Study the drawing (mm; zero at the part's minimum x, y, z) and answer. A direction names the side the tool comes from. Coordinates: 2 decimals unless noted, no trailing zeros. Order: outer loops, then holes, each group sorted by start corner. A loop starts at its lowest first (then second) coordinate and runs counter-clockwise, first axis right, second up. Notation, with made-up numbers: M 81,22.25 L 87,22.25 A14 ccw 87,46.25 Z; hole C 25,59.25 d2. An arc over 180 degrees is marked long. Use a Markdown table: item, result. Add a question column.
1) For the marked faces 1 and 2, determine the directions among +Z, -Z, +X, -X, +Y, -Y from which every point of the face is accessible in a straight line to the end or side of a thin tool.
2) Find section A-A on z = 14.5. Write down the section's boundary in (x, y) (1 decimal).
3) Find the intervals of material crossed by probe 1 along Y at (x, z) = (21, 4.5); probe 2 along X at (y, z) = (36.5, 2.25); probe 3 along Y at (x, z) = (11.5, 18.5), in increasing order. Write a range as [from, to].
4) Each of these flat-tipped pins is pushed along its axis until it touches: pin 1 Ø1.5 at (x, z) = (6.5, 3.5) entering from -Y (1 decimal); pin 2 Ø1.7 at (x, z) = (10, 9.5) entering from +Y; pin 3 Ø4 at (y, z) = (5.5, 17) entering from -X. Where does it stop, or does it pass through?
5) Find section B-B on x = 10. Write down the section's boundary in (y, z).
6) Find section C-C on y = 25.5. Write down the section's boundary in (x, z).
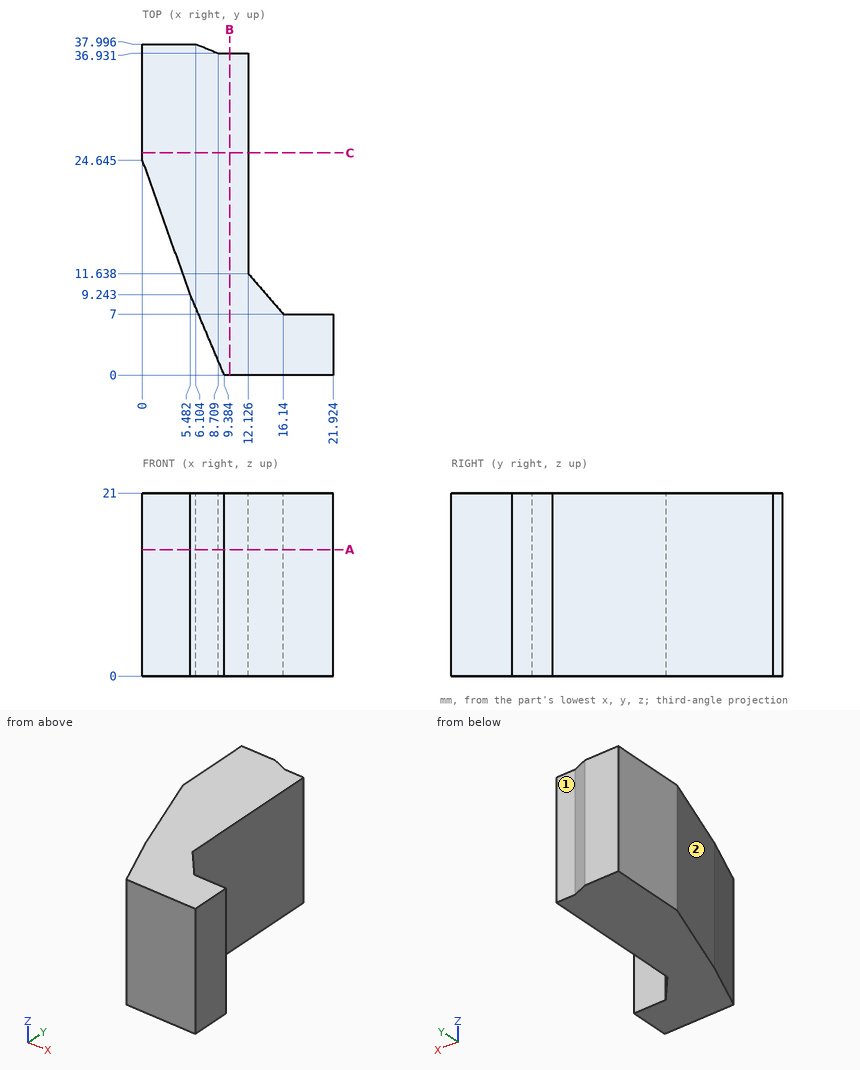
Check result:
| question | item | result |
|---|---|---|
| 1 | face 1 | +Z, -Z, +X, +Y |
| 1 | face 2 | +Z, -Z, -X, -Y |
| 2 | outline | M 0,24.6 L 5.5,9.2 L 9.4,0 L 21.9,0 L 21.9,7 L 16.1,7 L 12.1,11.6 L 12.1,36.9 L 8.7,36.9 L 6.1,38 L 0,38 Z |
| 3 | probe 1 | y = [0, 7] |
| 3 | probe 2 | x = [0, 12.13] |
| 3 | probe 3 | y = [0, 36.93] |
| 4 | pin 1 | stops at y = 5.1 |
| 4 | pin 2 | stops at y = 36.93 |
| 4 | pin 3 | stops at x = 6.22 |
| 5 | outline | M 0,0 L 36.93,0 L 36.93,21 L 0,21 Z |
| 6 | outline | M 0,0 L 12.13,0 L 12.13,21 L 0,21 Z |
